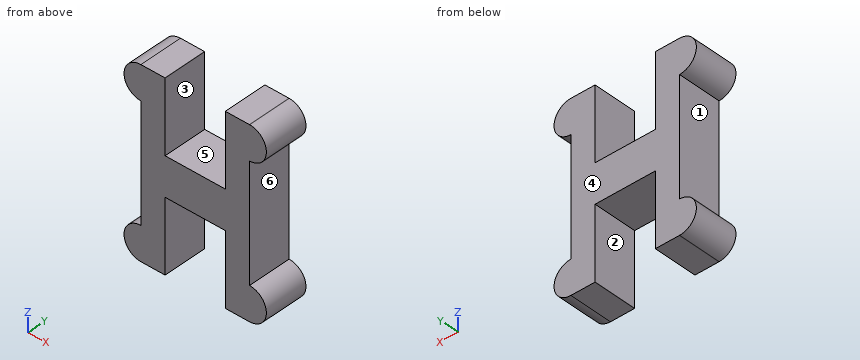
from build123d import *

# Parameters (mm, degrees)
SKETCH1_W           = 1
SKETCH1_H           = 1.4
BOSS_EXTRUDE1_DEPTH = 1.8


with BuildPart() as part:
    # Sketch1 → Boss-Extrude1 (new body)
    with BuildSketch(Plane(origin=(0, 0, 0), x_dir=(1, 0, 0), z_dir=(0, 1, 0))):
        Polygon((-2.25, 2.4), (-2.25, -2.4), (-1.25, -2.4), (-1.25, -0.8), (1.25, -0.8), (1.25, -2.4), (2.25, -2.4), (2.25, 2.4), (1.25, 2.4), (1.25, 0.8), (-1.25, 0.8), (-1.25, 2.4), align=None)
        with Locations((-1.75, 3.1)):
            Rectangle(SKETCH1_W, SKETCH1_H)
        with BuildLine():
            ThreePointArc((-2.25, 3.8), (-2.95, 3.1), (-2.25, 2.4))
            Line((-2.25, 2.4), (-2.25, 3.8))
        make_face()
        with Locations((1.75, 3.1)):
            Rectangle(SKETCH1_W, SKETCH1_H)
        with BuildLine():
            Line((2.25, 3.8), (2.25, 2.4))
            ThreePointArc((2.25, 2.4), (2.95, 3.1), (2.25, 3.8))
        make_face()
        with BuildLine():
            Line((2.25, -2.4), (2.25, -3.8))
            ThreePointArc((2.25, -3.8), (2.95, -3.1), (2.25, -2.4))
        make_face()
        with Locations((1.75, -3.1)):
            Rectangle(SKETCH1_W, SKETCH1_H)
        with Locations((-1.75, -3.1)):
            Rectangle(SKETCH1_W, SKETCH1_H)
        with BuildLine():
            ThreePointArc((-2.25, -2.4), (-2.95, -3.1), (-2.25, -3.8))
            Line((-2.25, -3.8), (-2.25, -2.4))
        make_face()
    extrude(amount=BOSS_EXTRUDE1_DEPTH)


solid = part.part
Geometry check sheet. Reference: the model listing, model coordinates, mm. Face numbers are marked on the shaded views. A direction names the side the tool comes from. Round coordinates to 2 decimals unless told otherwise and drop trailing zeros. Loops run counter-clockwise (first coordinate to the right, second up) from the corner with the lowest first, then second, coordinate; pieces in that order, holes last. Notation, with made-up numbers: (-23.5, -37.75) - (-17.5, -37.75) arc R17 cw to (-17.5, -14.75) - close; hole circle Ø9 at (-36, 0.25). An arc over 180 degrees is marked (long way). One line per question, with ' | ' between items. Start each with the question number.
1. Draft check along Z on the marked faces 4, 5 and 6. Enter one of: released by +Z, released by -Z, zero draft, split by the parting line, or undercut.
2. Cross-section at D-D on z = -0.5. Record the cut outline in (x, y).
3. Tool access check on the marked faces 1, 2 and 3. Record the directions out of +Z, -Z, +X, -X, +Y, -Y that give a thin tool (end or side, any length) a straight path to the whole face; none if there is none.
4. Cross-section at C-C on y = 0.95. Record the cut outline in (x, z), then the cut area to 3 significant figures.
5. Cross-section at B-B on x = -2.5. Record the cut outline in (y, z), then the cut area to 3 significant figures.
6. Depth check by flat-ended pin: pin 1 (0.5 mm diameter, centred on y = 1, z = 3, fed in from +X); pin 2 (1 mm diameter, centred on y = 0.5, z = 0, fed in from -X); pin 3 (0.5 mm diameter, centred on y = 1, z = 1, fed in from +X); pin 4 (0.9 mm diameter, centred on y = 1, z = 2.5, fed in from -X). Enter the tip coordinate at first touch or a pass-through.
7. Scan lines: line 1 (X direction, y = 1.4, z = 2.25); line 2 (Z direction, x = 0.3, y = 0.75); line 3 (Z direction, x = -2.3, y = 1.3). Record each from-to range of solid material in increasing order. Write a range as [from, to].
8. Cross-section at A-A on z = -3.1. Record the cut outline in (x, y).
Taken from the geometry:
1) face 4: zero draft | face 5: released by +Z | face 6: undercut
2) outline: (-2.25, 0) - (2.25, 0) - (2.25, 1.8) - (-2.25, 1.8) - close
3) face 1: -X, +Y, -Y | face 2: -Z, +Y, -Y | face 3: +Z, +Y, -Y
4) outline: (-2.25, -3.8) - (-1.25, -3.8) - (-1.25, -0.8) - (1.25, -0.8) - (1.25, -3.8) - (2.25, -3.8) arc R0.7 ccw to (2.25, -2.4) - (2.25, 2.4) arc R0.7 ccw to (2.25, 3.8) - (1.25, 3.8) - (1.25, 0.8) - (-1.25, 0.8) - (-1.25, 3.8) - (-2.25, 3.8) arc R0.7 ccw to (-2.25, 2.4) - (-2.25, -2.4) arc R0.7 ccw to start | area: 22.3 mm²
5) outline: (0, -3.75) - (1.8, -3.75) - (1.8, -2.45) - (0, -2.45) - close; (0, 2.45) - (1.8, 2.45) - (1.8, 3.75) - (0, 3.75) - close | area: 4.71 mm²
6) pin 1: x = 2.95 | pin 2: x = -2.25 | pin 3: x = 2.25 | pin 4: x = -2.93
7) line 1: [-2.25, -1.25], [1.25, 2.25] | line 2: [-0.8, 0.8] | line 3: [-3.8, -2.4], [2.4, 3.8]
8) outline: (-2.95, 0) - (-1.25, 0) - (-1.25, 1.8) - (-2.95, 1.8) - close; (1.25, 0) - (2.95, 0) - (2.95, 1.8) - (1.25, 1.8) - close
